Source: three-view drawing plus pictorial views. Frame: mm from the lowest corner of the part. A direction names the side the tool comes from. Coordinates: 2 decimals unless noted, no trailing zeros. Order: outer loops, then holes, each group sorted by start corner. A loop starts at its lowest first (then second) coordinate and runs counter-clockwise, first axis right, second up. Notation, with made-up numbers: (-19, 8.5) - (24, 8.5) arc R16 cw to (24, 15.5) - close; hole circle Ø5 at (-21.5, -19). An arc over 180 degrees is marked (long way). Use a Markdown table: item, result. Add a question column.
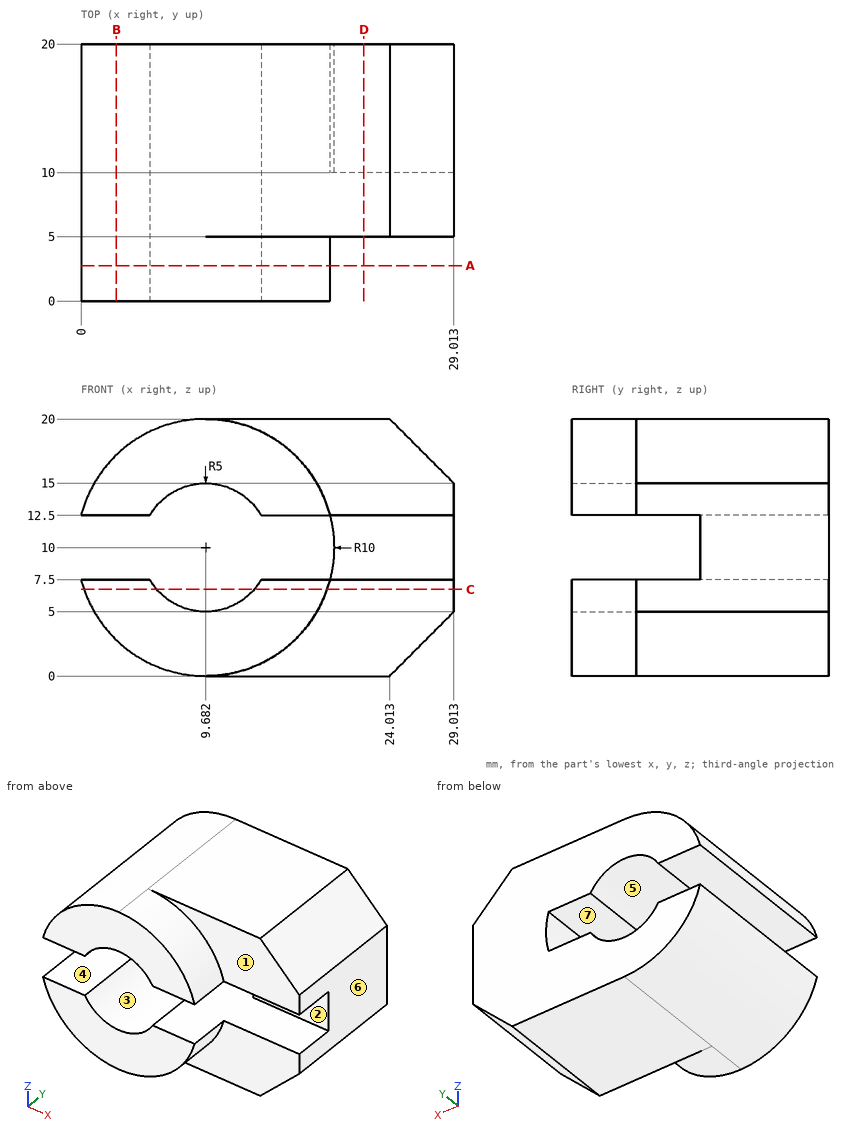
1) Section A-A (y = 2.75). Return loops of the section in (x, z) (1 decimal).
2) Section B-B (x = 2.75). Return loops of the section in (y, z), then the cut area to 3 significant figures.
3) Section C-C (z = 6.75). Return loops of the section in (x, y) (1 decimal).
4) Pin query (flat end, axial travel): pin 1 (3 mm diameter, centred on x = 4, y = 8.5, fed in from -Z); pin 2 (4.5 mm diameter, centred on x = 2, y = 7.5, fed in from -Z) (1 decimal); pin 3 (4.5 mm diameter, centred on x = 3.5, y = 8, fed in from +Z) (1 decimal). Return the tip coordinate at first contact, or that it passes through.
5) Set-up query: the marked faces 1, 2, 3 and 4. Return all of +Z, -Z, +X, -X, +Y, -Y with unobstructed straight access to the full face (end or side cutting, diameter ignored); none if empty.
6) Draft query along X for the marked faces 5, 6 and 7. Return one class per face: pulls with the +X half, pulls with the -X half, needs draft (parallel to the pull), parting line crosses it, or undercut.
7) Section D-D (x = 22). Return loops of the section in (y, z).
8) Ray query, line 1 along Z through (x, y) = (17.75, 15); line 2 along Z through (x, y) = (9.5, 19); line 3 along X through (y, z) = (14, 9.75). Return the intervals inside material, ascending.
Values follow:
| question | item | result |
|---|---|---|
| 1 | outline | (0, 7.5) arc R10 ccw to (9.7, 0) arc R10 ccw to (19.4, 7.5) - (14, 7.5) arc R5 cw to (5.4, 7.5) - close; (0, 12.5) - (5.4, 12.5) arc R5 cw to (14, 12.5) - (19.4, 12.5) arc R10 ccw to (9.7, 20) arc R10 ccw to start |
| 2 | outline | (0, 2.79) - (20, 2.79) - (20, 7.5) - (0, 7.5) - close; (0, 12.5) - (20, 12.5) - (20, 17.21) - (0, 17.21) - close |
| 2 | area | 188 mm² |
| 3 | outline | (0.2, 0) - (5.9, 0) - (5.9, 20) - (0.2, 20) - close; (13.5, 0) - (19.1, 0) - (19.1, 5) - (29, 5) - (29, 20) - (13.5, 20) - close |
| 4 | pin 1 | stops at z = 0.92 |
| 4 | pin 2 | stops at z = 1.6 |
| 4 | pin 3 | stops at z = 19.2 |
| 5 | face 1 | +Z, +X, -Y |
| 5 | face 2 | +X, -X, -Y |
| 5 | face 3 | +Y, -Y |
| 5 | face 4 | -X, +Y, -Y |
| 6 | face 5 | undercut |
| 6 | face 6 | pulls with the +X half |
| 6 | face 7 | needs draft |
| 7 | outline | (5, 0) - (20, 0) - (20, 20) - (5, 20) - (5, 12.5) - (10, 12.5) - (10, 7.5) - (5, 7.5) - close |
| 8 | line 1 | z = 0 to 7.5, 12.5 to 20 |
| 8 | line 2 | z = 0 to 5, 15 to 20 |
| 8 | line 3 | x = 19.68 to 29.01 |
